CAD build for the part. Positions are in the model's coordinates, mm. Give positions to 0.01 mm unless a question says otherwise; leave off trailing zeros. Write each loop counter-clockwise with the first axis right and the second up, starting at its lowest first coordinate (ties: lowest second). Pieces come first, ordered by that corner, then holes. Notation, with made-up numbers: (-5.5, -26) - (35.5, -26) arc R35 cw to (35.5, 11) - close; hole circle Ø5 at (23, 4). An arc over 180 degrees is marked (long way). Answer as a JSON object with one key per item and string values.
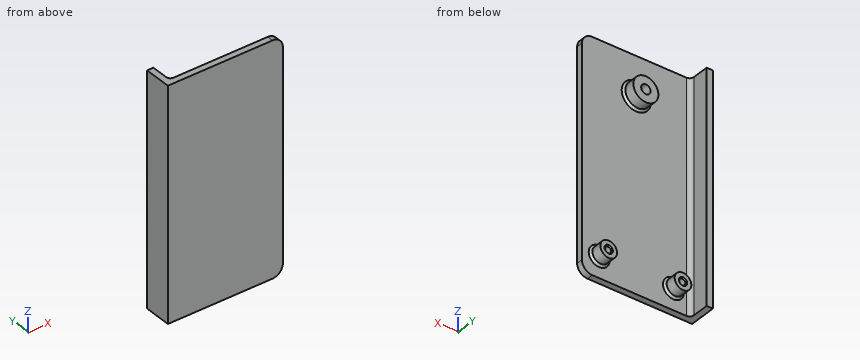
Autodesk Inventor part; units mm, degrees
ref_plane "YZ Plane" through (0, 0, 0) normal (1, 0, 0) x (0, 1, 0)
ref_plane "XZ Plane" through (0, 0, 0) normal (0, 1, 0) x (-1, 0, 0)
ref_plane "XY Plane" through (0, 0, 0) normal (0, 0, 1) x (1, 0, 0)
sketch "Sketch1" plane through (0, 0, 0) normal (0, 1, 0) x (-1, 0, 0)
  line L0 (0, 0) -> (-55.1, 0)
  line L1 (-55.1, 0) -> (-55.1, -110)
  line L2 (-55.1, -110) -> (0, -110)
  line L3 (0, -110) -> (0, 0)
  dimension "d0" = 110
  dimension "d28" = 55.1
extrude "Extrusion1" add sketch "Sketch1" along normal blind 3
sketch "Sketch2" plane through (0, 3, 0) normal (0, 1, 0) x (1, 0, 0)
  line L0 (55.1, 0) -> (55.1, 110)
  line L1 (55.1, 110) -> (0, 110)
  line L2 (0, 110) -> (0, 0)
  line L3 (0, 0) -> (55.1, 0)
  circle A0 centre (11.25, 99.95) radius 4
  circle A1 centre (46.85, 99.95) radius 4
  circle A2 centre (29.05, 18.6623) radius 6
  point P0 (27.55, 110)
  dimension "d3" = 8
  dimension "d4" = 10.05
  dimension "d6" = 8
  dimension "d7" = 10.05
  dimension "d8" = 8.25
  dimension "d29" = 12
  dimension "d30" = 91.35
  dimension "d39" = 26.05
  dimension "d40" = 35.6
extrude "Extrusion2" cut sketch "Sketch2" against normal blind 0.5 contours A0 | A1 | A2
sketch "Sketch3" plane through (11.25, 2.5, -99.95) normal (0, 1, 0) x (1, 0, 0)
  circle A0 centre (0, 0) radius 4
  circle A1 centre (0, 0) radius 4
  circle A2 centre (35.6, 0) radius 4
  circle A3 centre (35.6, 0) radius 4
  circle A4 centre (17.8, -81.2877) radius 6
  circle A5 centre (17.8, -81.2877) radius 6
  point P0 (-11.25, -99.95)
  dimension "d32" = 12
extrude "Extrusion3" add sketch "Sketch3" along normal blind 6.5
sketch "Sketch4" plane through (11.25, 9, -99.95) normal (0, 1, 0) x (1, 0, 0)
  circle A0 centre (0, 0) radius 4
  circle A1 centre (0, 0) radius 1.5
  circle A2 centre (35.6, 0) radius 4
  circle A3 centre (35.6, 0) radius 1.5
  point P0 (-11.25, -99.95)
  dimension "d13" = 3
  dimension "d14" = 3
extrude "Extrusion4" cut sketch "Sketch4" against normal blind 3.7 contours A1 | A3
chamfer "Chamfer1" distance 1 angle 45 3 edges at (7.25, 3, -99.95) (42.85, 3, -99.95) (23.05, 3, -18.6623)
chamfer "Chamfer2" distance 0.5 angle 45 2 edges at (9.75, 9, -99.95) (45.35, 9, -99.95)
sketch "Sketch5" plane through (0, 3, 0) normal (0, 1, 0) x (1, 0, 0)
  circle A0 centre (11.25, 99.95) radius 1.5
  point P0 (0, 0)
sketch "Sketch6" plane through (11.25, 5.3, -99.95) normal (0, 1, 0) x (1, 0, 0)
  circle A0 centre (0, 0) radius 1.5
  circle A1 centre (0, 0) radius 1.1
  circle A2 centre (35.6, 0) radius 1.5
  circle A3 centre (35.6, 0) radius 1.1
  point P0 (-11.25, -99.95)
  dimension "d23" = 2.2
  dimension "d24" = 2.2
extrude "Extrusion5" cut sketch "Sketch6" against normal blind 1.3 contours A1 | A3
sketch "Sketch7" plane through (29.05, 9, -18.6623) normal (0, 1, 0) x (1, 0, 0)
  circle A0 centre (0, 0) radius 2.25
  point P0 (-29.05, -18.6623)
  dimension "d33" = 4.5
extrude "Extrusion6" cut sketch "Sketch7" against normal blind 4.2
sketch "Sketch8" plane through (29.05, 4.8, -18.6623) normal (0, 1, 0) x (1, 0, 0)
  circle A0 centre (0, 0) radius 2.25
  circle A1 centre (0, 0) radius 1.6
  point P0 (-29.05, -18.6623)
  dimension "d36" = 3.2
extrude "Extrusion7" cut sketch "Sketch8" against normal blind 1.8 contours A1
sketch "Sketch9" plane through (0, 3, 0) normal (0, 1, 0) x (1, 0, 0)
  circle A0 centre (46.85, 99.95) radius 5
  line L0 (55.1, 0) -> (55.1, 110)
  line L1 (55.1, 110) -> (0, 110)
  line L2 (0, 110) -> (0, 0)
  line L3 (0, 0) -> (55.1, 0)
  circle A1 centre (11.25, 99.95) radius 5
  circle A2 centre (29.05, 18.6623) radius 7
  line L4 (55.1, 110) -> (0, 110)
  line L5 (0, 110) -> (3, 110)
  line L6 (3, 110) -> (3, 0)
  line L7 (3, 0) -> (0, 0)
  line L8 (0, 0) -> (0, 110)
  dimension "d41" = 3
extrude "Extrusion8" add sketch "Sketch9" along normal blind 10 contours L3 L2 L1 L6
fillet "Fillet2" radius 5 2 edges at (55.1, 1.5, -110) (55.1, 1.5, 0)
fillet "Fillet3" radius 2 1 edges at (3, 3, -55)
properties part number "long_protoboard_backplate"
(1) Saw through at A-A, the plane z = -48. Give the cut face in (x, y), and give its area (3 significant figures).
Answer key:
{"outline": "(0, 0) - (55.1, 0) - (55.1, 3) - (5, 3) arc R2 cw to (3, 5) - (3, 13) - (0, 13) - close", "area": "196 mm²"}
(2) Saw through at D-D, the plane x = 40. Give the cut face in (y, z).
Answer key:
{"outline": "(0, -110) - (3, -110) - (3, 0) - (0, 0) - close"}
(3) Probe L1, parallel to Z at x = 46.85, y = 7.7; L2, parallel to X at y = 6.5, z = -102; L3, parallel to X at y = 4.3, z = -99.95. List the from-to ranges inside material, lowest first. Write a range as [from, to].
Answer key:
{"L1": "z = [-103.95, -101.45], [-98.45, -95.95]", "L2": "x = [0, 3], [7.82, 14.68], [43.42, 50.28]", "L3": "x = [0, 3.13], [7.25, 10.15], [12.35, 15.25], [42.85, 45.75], [47.95, 50.85]"}
(4) Flat gauge pins, fed straight in: P1, Ø1.3, axis at x = 46.85, z = -99.95, coming from the +Y side; P2, Ø2.5, axis at y = 8.5, z = -65.5, coming from the +X side; P3, Ø1.5, axis at x = 47.5, z = -100.5, coming from the +Y side. Where does each tip first touch, or does it go through?
Answer key:
{"P1": "stops at y = 4", "P2": "stops at x = 3", "P3": "stops at y = 8.6"}
(5) Saw through at C-C, the plane x = 46.85. Give the cut face in (y, z).
Answer key:
{"outline": "(0, -110) - (3, -110) - (3, -104.95) - (4, -103.95) - (9, -103.95) - (9, -101.95) - (8.5, -101.45) - (5.3, -101.45) - (5.3, -101.05) - (4, -101.05) - (4, -98.85) - (5.3, -98.85) - (5.3, -98.45) - (8.5, -98.45) - (9, -97.95) - (9, -95.95) - (4, -95.95) - (3, -94.95) - (3, 0) - (0, 0) - close"}
(6) Saw through at B-B, the plane x = 29.05. Give the cut face in (y, z), and give its area (3 significant figures).
Answer key:
{"outline": "(0, -110) - (3, -110) - (3, -25.66) - (4, -24.66) - (9, -24.66) - (9, -20.91) - (4.8, -20.91) - (4.8, -20.26) - (3, -20.26) - (3, -17.06) - (4.8, -17.06) - (4.8, -16.41) - (9, -16.41) - (9, -12.66) - (4, -12.66) - (3, -11.66) - (3, 0) - (0, 0) - close", "area": "378 mm²"}
